from build123d import *

# Parameters (mm, degrees)
F1_DEPTH = 165.1
F3_W     = 120.2936734515
F3_H     = 44.45
F4_DEPTH = 6.35
F6_W     = 105.5140421895
F6_H     = 44.45
F7_DEPTH = 6.35


with BuildPart() as f1:
    # F0 (on Front) → F1 (new body)
    with BuildSketch(Plane.XZ):
        with BuildLine():
            ThreePointArc((55.2767035972, 50.8), (67.8600718832, 26.4462179087), (75.0743229112, 0))
            Line((75.0743229112, 0), (96.4022464211, 0))
            Line((96.4022464211, 0), (96.4022464211, 50.8))
            Line((96.4022464211, 50.8), (55.2767035972, 50.8))
        make_face()
    extrude(amount=F1_DEPTH)

    # F3 (on offset) → F4 (cut)
    with BuildSketch(Plane.XZ.offset(139.7)):
        with Locations((60.1468367257, 22.225)):
            Rectangle(F3_W, F3_H)
    extrude(amount=-F4_DEPTH, mode=Mode.SUBTRACT)

    # F6 (on offset) → F7 (cut)
    with BuildSketch(Plane(origin=(0, -25.4, 0), x_dir=(-1, 0, 0), z_dir=(0, 1, 0))):
        with Locations((-52.7570210947, 22.225)):
            Rectangle(F6_W, F6_H)
    extrude(amount=-F7_DEPTH, mode=Mode.SUBTRACT)


solid = f1.part
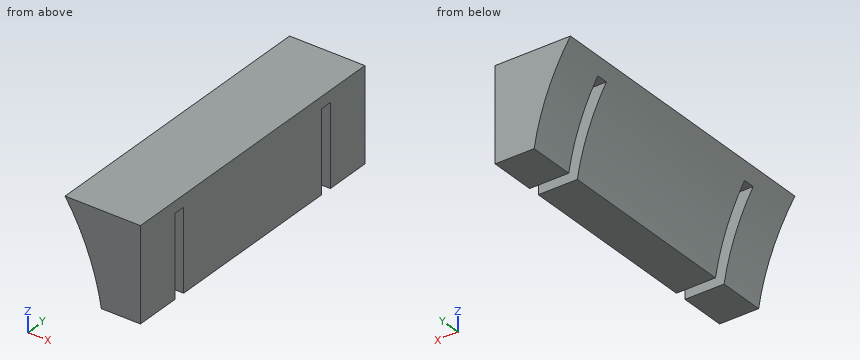
Design review of the part built by this model. Coordinates are the model's own, in mm. Give positions to 0.01 mm unless a question says otherwise; leave off trailing zeros. Loops run counter-clockwise (first coordinate to the right, second up) from the corner with the lowest first, then second, coordinate; pieces in that order, holes last. Notation, with made-up numbers: M 36.5,84 L 83.5,84 A28 cw 83.5,120 Z; hole C -13,-9 d2. An arc over 180 degrees is marked long. Write item = value, one per line.
Q1. We need section B-B (x = 89.5). Give the boundary of the cut face in (y, z).
Output values:
outline = M -165.1,0 L -139.7,0 L -139.7,44.45 L -133.35,44.45 L -133.35,0 L -31.75,0 L -31.75,44.45 L -25.4,44.45 L -25.4,0 L 0,0 L 0,50.8 L -165.1,50.8 Z
Q2. We need section A-A (z = 36). Give the boundary of the cut face in (x, y).
Output values:
outline = M 63.69,-165.1 L 96.4,-165.1 L 96.4,-139.7 L 63.69,-139.7 Z; M 63.69,-133.35 L 96.4,-133.35 L 96.4,-31.75 L 63.69,-31.75 Z; M 63.69,-25.4 L 96.4,-25.4 L 96.4,0 L 63.69,0 Z
Q3. To check wall thickness, follow line 1 (Y direction, x = 73, z = 34); line 2 (Z direction, x = 71, y = -28); line 3 (Z direction, x = 67, y = -69). State the ranges of each line that lie inside material, in increasing order. Write a range as [from, to].
Output values:
line_1 = [-165.1, -139.7], [-133.35, -31.75], [-25.4, 0]
line_2 = [44.45, 50.8]
line_3 = [28.6, 50.8]
Q4. We need section C-C (z = 6.5). Give the boundary of the cut face in (x, y).
Output values:
outline = M 73.85,-165.1 L 96.4,-165.1 L 96.4,-139.7 L 73.85,-139.7 Z; M 73.85,-133.35 L 96.4,-133.35 L 96.4,-31.75 L 73.85,-31.75 Z; M 73.85,-25.4 L 96.4,-25.4 L 96.4,0 L 73.85,0 Z
Q5. Insertion check: pin 1 (1.5 mm diameter, centred on y = -146, z = 32, fed in from -X); pin 2 (5 mm diameter, centred on x = 71.5, y = -28.5, fed in from -Z); pin 3 (1 mm diameter, centred on y = -98, z = 30.5, fed in from -X). Each pin has a flat end and moves straight along its axis. Give the tip position at first contact, or say it passes through.
Output values:
pin_1 = 65.21
pin_2 = 44.45
pin_3 = 65.99
Q6. We need section D-D (y = -93). Give the boundary of the cut face in (x, z).
Output values:
outline = M 55.28,50.8 A130.4 cw 75.07,0 L 96.4,0 L 96.4,50.8 Z
